from build123d import *

# Parameters (mm, degrees)
SKETCH1_W            = 63.5
SKETCH1_H            = 203.2
BOSS_EXTRUDE1_DEPTH  = 12.7
SKETCH2_R            = 3.175
CUT_EXTRUDE1_DEPTH   = 108.200338152
LPATTERN1_COUNT      = 2
LPATTERN1_PITCH      = 38.1
LPATTERN1_COUNT_DIR2 = 2
LPATTERN1_PITCH_DIR2 = 177.8
SKETCH3_R            = 20.6375
CUT_EXTRUDE2_DEPTH   = 108.200338152


with BuildPart() as part:
    # Sketch1 → Boss-Extrude1 (new body)
    with BuildSketch(Plane.XY):
        Rectangle(SKETCH1_W, SKETCH1_H)
    extrude(amount=BOSS_EXTRUDE1_DEPTH)

    # Sketch2 → Cut-Extrude1 (cut, through all)
    with BuildSketch(Plane.XY.offset(12.7)):
        with Locations((-19.05, 88.9)):
            Circle(SKETCH2_R)
    cut_extrude1 = extrude(amount=-CUT_EXTRUDE1_DEPTH, mode=Mode.SUBTRACT)

    # LPattern1: Cut-Extrude1 2 × 2
    with Locations(*[(i * LPATTERN1_PITCH, -j * LPATTERN1_PITCH_DIR2, 0) for i in range(LPATTERN1_COUNT) for j in range(LPATTERN1_COUNT_DIR2) if (i, j) != (0, 0)]):
        add(cut_extrude1, mode=Mode.SUBTRACT)

    # Sketch3 → Cut-Extrude2 (cut, through all)
    with BuildSketch(Plane.XY.offset(12.7)):
        with Locations((0, -12.7)):
            Circle(SKETCH3_R)
    extrude(amount=-CUT_EXTRUDE2_DEPTH, mode=Mode.SUBTRACT)


solid = part.part
Input: part model. Units: mm. Frame: model coordinates. Give positions to 0.01 mm unless a question says otherwise; leave off trailing zeros. Write each loop counter-clockwise with the first axis right and the second up, starting at its lowest first coordinate (ties: lowest second). Pieces come first, ordered by that corner, then holes. Notation, with made-up numbers: M -0.5,-21 L 49.5,-21 A11 ccw 49.5,-5 Z; hole C 71.5,89.25 d7. An arc over 180 degrees is marked long. Write item = value, one per line. Start each with the question number.
1) Cut plane D-D on y = -12.7. Return the cut outline in (x, z).
2) Cut plane B-B on x = 0. Return the cut outline in (y, z), then the cut area to 3 significant figures.
3) Cut plane C-C on z = 6.5. Count the separate pieces of the cut face and the enclosed holes in it, then the cut area to 3 significant figures.
4) Draft query along X for faces 1 (the cylindrical face through (-19.74, 85.8, 6.44)), 2 (the flat face through (0, -101.6, 6)), 3 (the cylindrical face through (-17.343, -86.223, 6.439)), 4 (the flat face through (31.75, -1, 6)). Return one class per face: +X half, -X half, draft (parallel to the pull), parting line (faces both ways), or undercut.
5) Cut plane A-A on y = 88.9. Return the cut outline in (x, z) (3 decimals), then the cut area to 3 significant figures.
6) Material intervals for line 1 along Y through (x, z) = (1, 7.5); line 2 along Y through (x, z) = (19.05, 10.25) (1 decimal); line 3 along Y through (x, z) = (15.5, 10.25), sorted ascending. Write a range as [from, to].
Solved:
q1.outline = M -31.75,0 L -20.64,0 L -20.64,12.7 L -31.75,12.7 Z; M 20.64,0 L 31.75,0 L 31.75,12.7 L 20.64,12.7 Z
q2.outline = M -101.6,0 L -33.34,0 L -33.34,12.7 L -101.6,12.7 Z; M 7.94,0 L 101.6,0 L 101.6,12.7 L 7.94,12.7 Z
q2.area = 2,060 mm2
q3.separate_pieces = 1
q3.enclosed_holes = 5
q3.area = 11,400 mm2
q4.face_1 = undercut
q4.face_2 = draft
q4.face_3 = undercut
q4.face_4 = +X half
q5.outline = M -31.75,0 L -22.225,0 L -22.225,12.7 L -31.75,12.7 Z; M -15.875,0 L 15.875,0 L 15.875,12.7 L -15.875,12.7 Z; M 22.225,0 L 31.75,0 L 31.75,12.7 L 22.225,12.7 Z
q5.area = 645 mm2
q6.line_1 = [-101.6, -33.31], [7.91, 101.6]
q6.line_2 = [-101.6, -92.1], [-85.7, -20.6], [-4.8, 85.7], [92.1, 101.6]
q6.line_3 = [-101.6, -26.33], [0.93, 101.6]
